Here's how the part is built. I have some questions about the finished solid (model axes, mm). Face numbers are marked on the shaded views. A direction names the side the tool comes from. Give positions to 0.01 mm unless a question says otherwise; leave off trailing zeros. Order: outer loops, then holes, each group sorted by start corner. A loop starts at its lowest first (then second) coordinate and runs counter-clockwise, first axis right, second up. Notation, with made-up numbers: (24, 35) -> (35, 35) arc R28 ccw to (35, 61) -> close; hole circle Ø7 at (46, -29). An arc over 180 degrees is marked (long way). Write each question's results on one line, items separated by ' | '. Start each with the question number.
Q1. Imagine slicing it at D-D, the plane x = 10.75. Please give me the cut outline in (y, z), then the cut area to 3 significant figures.
Q2. Imagine slicing it at B-B, the plane z = 21. Please give me the cut outline in (x, y).
Q3. Imagine slicing it at C-C, the plane x = 15. Please give me the cut outline in (y, z).
Q4. For the marked faces 4, 5 and 6, which set-ups out of +Z, -Z, +X, -X, +Y, -Y let a thin tool reach every point of the face, with its end or its side?
Q5. I'm going to push flat-ended pins straight in: pin 1 (1.5 mm diameter, centred on y = -6.5, z = 3.5, fed in from -X); pin 2 (5 mm diameter, centred on x = 12.5, z = 23, fed in from +Y); pin 3 (3 mm diameter, centred on y = -3, z = 16.5, fed in from -X). Where does each tip first touch, or does it pass through?
Q6. I need wall thicknesses on line 1 along X through (y, z) = (19.5, 12); line 2 along X through (y, z) = (-10.5, 11); line 3 along Y through (x, z) = (20.75, 27.5). Which ranges of each line are inside material? Lowest first, please. Write a range as [from, to].
Q7. Thinking about a two-plate mould opening in X: for the marked faces 1, 2 and 3, which applies, pulls with the +X half, pulls with the -X half, needs draft (parallel to the pull), parting line crosses it, or undercut?
Q8. Imagine slicing it at A-A, the plane y = 18.5. Please give me the cut outline in (x, z), then the cut area to 3 significant figures.
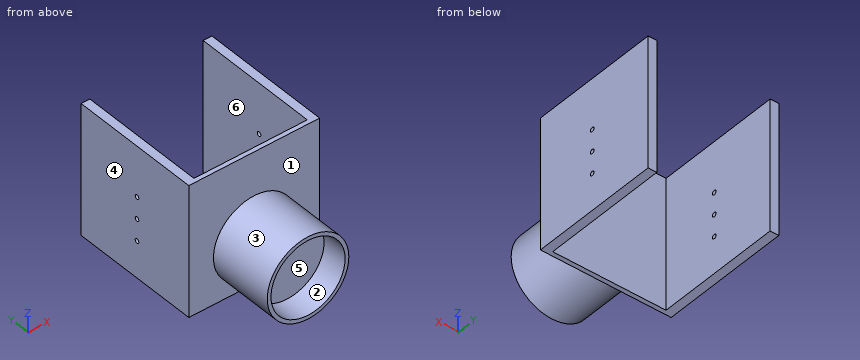
```python
from build123d import *

# Parameters (mm, degrees)
BOSS_EXTRUDE2_DEPTH = 30
SKETCH2_R           = 9.357027653
BOSS_EXTRUDE3_DEPTH = 15
SKETCH3_R           = 8.504853576
CUT_EXTRUDE1_DEPTH  = 5.87
SKETCH4_R           = 0.5
CUT_EXTRUDE2_DEPTH  = 37.592


with BuildPart() as part:
    # Sketch1 → Boss-Extrude2 (new body)
    with BuildSketch(Plane.XY):
        Polygon((0, 30), (0, 0), (30, 0), (30, 30), (28, 30), (28, 1), (1.999996, 1), (1.999996, 30), align=None)
    extrude(amount=BOSS_EXTRUDE2_DEPTH)

    # Sketch2 → Boss-Extrude3 (add)
    with BuildSketch(Plane.XZ):
        with Locations((15, 10.669629744)):
            Circle(SKETCH2_R)
    extrude(amount=BOSS_EXTRUDE3_DEPTH)

    # Sketch3 → Cut-Extrude1 (cut)
    with BuildSketch(Plane.XZ.offset(15)):
        with Locations((15, 10.669629744)):
            Circle(SKETCH3_R)
    extrude(amount=-CUT_EXTRUDE1_DEPTH, mode=Mode.SUBTRACT)

    # Sketch4 → Cut-Extrude2 (cut)
    with BuildSketch(Plane.ZY):
        with Locations(Location((8.409330375, 14.442206742, 0), (0, 0, 270))):
            Circle(SKETCH4_R)
        with Locations(Location((13.409330375, 14.442206742, 0), (0, 0, 270))):
            Circle(SKETCH4_R)
        with Locations(Location((18.409330375, 14.442206742, 0), (0, 0, 270))):
            Circle(SKETCH4_R)
    extrude(amount=-CUT_EXTRUDE2_DEPTH, mode=Mode.SUBTRACT)


solid = part.part
```
Geometry check:
1) outline: (-15, 2.33) -> (0, 2.33) -> (0, 0) -> (1, 0) -> (1, 30) -> (0, 30) -> (0, 19.01) -> (-15, 19.01) -> (-15, 18.04) -> (-9.13, 18.04) -> (-9.13, 3.3) -> (-15, 3.3) -> close | area: 194 mm²
2) outline: (0, 0) -> (30, 0) -> (30, 30) -> (28, 30) -> (28, 1) -> (2, 1) -> (2, 30) -> (0, 30) -> close
3) outline: (-15, 1.31) -> (0, 1.31) -> (0, 0) -> (1, 0) -> (1, 30) -> (0, 30) -> (0, 20.03) -> (-15, 20.03) -> (-15, 19.17) -> (-9.13, 19.17) -> (-9.13, 2.16) -> (-15, 2.16) -> close
4) face 4: +Z, -Z, -X, +Y, -Y | face 5: -Y | face 6: +Z, -Z, +Y
5) pin 1: x = 8.19 | pin 2: y = 1 | pin 3: x = 6.71
6) line 1: [0, 2], [28, 30] | line 2: [5.65, 6.5], [23.5, 24.35] | line 3: [0, 1]
7) face 1: needs draft | face 2: undercut | face 3: parting line crosses it
8) outline: (0, 0) -> (2, 0) -> (2, 30) -> (0, 30) -> close; (28, 0) -> (30, 0) -> (30, 30) -> (28, 30) -> close | area: 120 mm²
